Check sheet for the drawn part. Datum: minimum x, y, z corner. Units: mm. Coordinates: 2 decimals unless noted, no trailing zeros. Write each loop counter-clockwise with the first axis right and the second up, starting at its lowest first coordinate (ties: lowest second). Pieces come first, ordered by that corner, then holes. Notation, with made-up numbers: M 0.25,-37 L 35.25,-37 A23 cw 35.25,-27 Z; hole C 23.5,42.25 d2. An arc over 180 degrees is marked long. Answer in a Markdown table with one row per item.
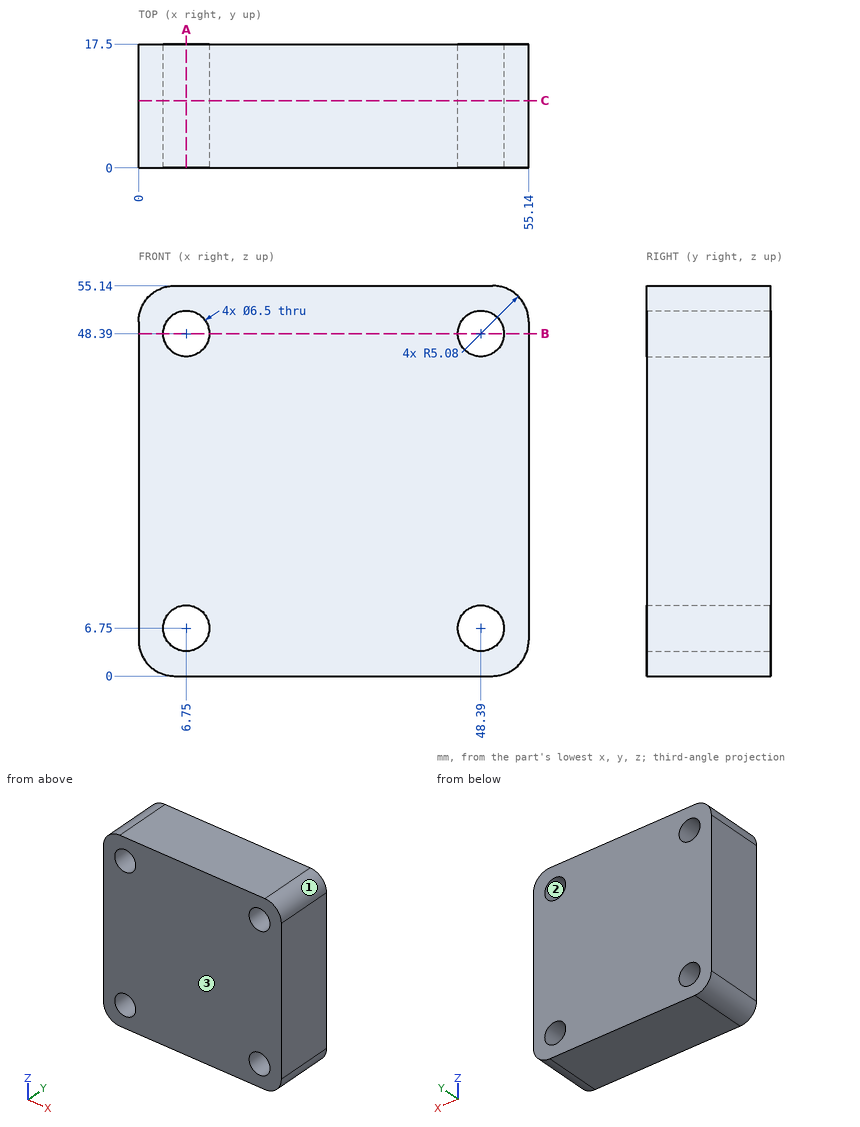
1) Depth check by flat-ended pin: pin 1 (8.5 mm diameter, centred on x = 6.75, z = 6.75, fed in from -Y). Enter the tip coordinate at first touch or a pass-through.
Response values:
| item | result |
|---|---|
| pin 1 | stops at y = 0 |
2) Sectioned sample at A-A (x = 6.75). Record the cut outline in (y, z).
Response values:
| item | result |
|---|---|
| outline | M 0,0 L 17.5,0 L 17.5,3.5 L 0,3.5 Z; M 0,10 L 17.5,10 L 17.5,45.14 L 0,45.14 Z; M 0,51.64 L 17.5,51.64 L 17.5,55.14 L 0,55.14 Z |
3) Sectioned sample at C-C (y = 9.5). Record the cut outline in (x, z).
Response values:
| item | result |
|---|---|
| outline | M 0,5.08 A5.08 ccw 5.08,0 L 50.06,0 A5.08 ccw 55.14,5.08 L 55.14,50.06 A5.08 ccw 50.06,55.14 L 5.08,55.14 A5.08 ccw 0,50.06 Z; hole C 6.75,6.75 d6.5; hole C 6.75,48.39 d6.5; hole C 48.39,6.75 d6.5; hole C 48.39,48.39 d6.5 |
4) Release check for a two-part mould opening along X. For the marked faces 1, 2 and 3 record: +X half, -X half, draft (parallel to the pull), parting line (faces both ways), or undercut.
Response values:
| item | result |
|---|---|
| face 1 | +X half |
| face 2 | undercut |
| face 3 | draft |
5) Sectioned sample at B-B (z = 48.39). Record the cut outline in (x, y), then the cut area to 3 significant figures.
Response values:
| item | result |
|---|---|
| outline | M 0,0 L 3.5,0 L 3.5,17.5 L 0,17.5 Z; M 10,0 L 45.14,0 L 45.14,17.5 L 10,17.5 Z; M 51.64,0 L 55.14,0 L 55.14,17.5 L 51.64,17.5 Z |
| area | 737 mm² |
6) Thickness scan on L1, parallel to X at y = 9.5, z = 48.39; L2, parallel to Z at x = 51, y = 5.75. Record the ranges inside material, lowest first. Write a range as [from, to].
Response values:
| item | result |
|---|---|
| L1 | x = [0, 3.5], [10, 45.14], [51.64, 55.14] |
| L2 | z = [0.09, 4.81], [8.69, 46.45], [50.33, 55.05] |
